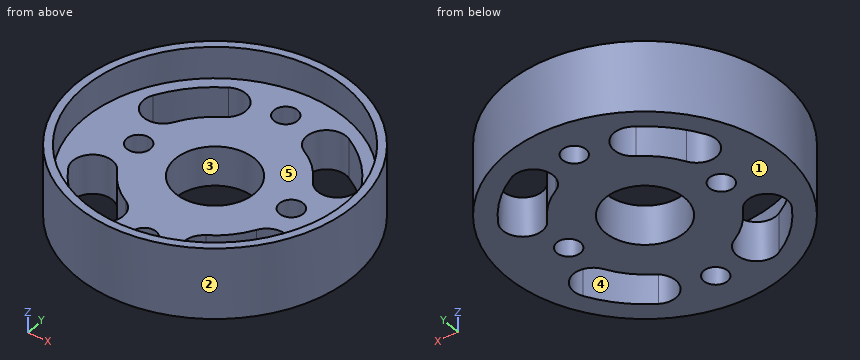
from build123d import *

# Parameters (mm, degrees)
SKETCH1_R           = 17.5
SKETCH1_R_2         = 1.5
SKETCH1_R_3         = 5
BOSS_EXTRUDE1_DEPTH = 5
SKETCH2_R           = 17.5
SKETCH2_R_2         = 16.5
EXTRUDE_THIN1_DEPTH = 4


with BuildPart() as part:
    # Sketch1 → Boss-Extrude1 (new body)
    with BuildSketch(Plane.XY):
        Circle(SKETCH1_R)
        with Locations((0, 12.5)):
            Circle(SKETCH1_R_2, mode=Mode.SUBTRACT)
        with Locations((0, -12.5)):
            Circle(SKETCH1_R_2, mode=Mode.SUBTRACT)
        Circle(SKETCH1_R_3, mode=Mode.SUBTRACT)
        with Locations((9.5, 0)):
            Circle(SKETCH1_R_2, mode=Mode.SUBTRACT)
        with Locations((-9.5, 0)):
            Circle(SKETCH1_R_2, mode=Mode.SUBTRACT)
        with BuildLine():
            ThreePointArc((-8.660254038, -5), (-7.071067812, -7.071067812), (-5, -8.660254038))
            ThreePointArc((-5, -8.660254038), (-4.084936491, -12.075317547), (-7.5, -12.990381057))
            ThreePointArc((-7.5, -12.990381057), (-10.606601718, -10.606601718), (-12.990381057, -7.5))
            ThreePointArc((-12.990381057, -7.5), (-12.075317547, -4.084936491), (-8.660254038, -5))
        make_face(mode=Mode.SUBTRACT)
        with BuildLine():
            ThreePointArc((-5, 8.660254038), (-4.084936491, 12.075317547), (-7.5, 12.990381057))
            ThreePointArc((-7.5, 12.990381057), (-10.606601718, 10.606601718), (-12.990381057, 7.5))
            ThreePointArc((-12.990381057, 7.5), (-12.075317547, 4.084936491), (-8.660254038, 5))
            ThreePointArc((-8.660254038, 5), (-7.071067812, 7.071067812), (-5, 8.660254038))
        make_face(mode=Mode.SUBTRACT)
        with BuildLine():
            ThreePointArc((5, -8.660254038), (4.084936491, -12.075317547), (7.5, -12.990381057))
            ThreePointArc((7.5, -12.990381057), (10.606601718, -10.606601718), (12.990381057, -7.5))
            ThreePointArc((12.990381057, -7.5), (12.075317547, -4.084936491), (8.660254038, -5))
            ThreePointArc((8.660254038, -5), (7.071067812, -7.071067812), (5, -8.660254038))
        make_face(mode=Mode.SUBTRACT)
        with BuildLine():
            ThreePointArc((12.990381057, 7.5), (12.075317547, 4.084936491), (8.660254038, 5))
            ThreePointArc((8.660254038, 5), (7.071067812, 7.071067812), (5, 8.660254038))
            ThreePointArc((5, 8.660254038), (4.084936491, 12.075317547), (7.5, 12.990381057))
            ThreePointArc((7.5, 12.990381057), (10.606601718, 10.606601718), (12.990381057, 7.5))
        make_face(mode=Mode.SUBTRACT)
    extrude(amount=BOSS_EXTRUDE1_DEPTH)

    # Sketch2 → Extrude-Thin1 (add)
    with BuildSketch(Plane.XY.offset(5)):
        Circle(SKETCH2_R)
        Circle(SKETCH2_R_2, mode=Mode.SUBTRACT)
    extrude(amount=EXTRUDE_THIN1_DEPTH)


solid = part.part
Can you work these out from the model? Positions are in its coordinate system, mm. Face numbers are marked on the shaded views. A direction names the side the tool comes from. Round coordinates to 2 decimals unless told otherwise and drop trailing zeros. Loops run counter-clockwise (first coordinate to the right, second up) from the corner with the lowest first, then second, coordinate; pieces in that order, holes last. Notation, with made-up numbers: (9.5, 37) - (63.5, 37) arc R29 cw to (63.5, 74) - close; hole circle Ø6 at (8, -21.5). An arc over 180 degrees is marked (long way). Answer in a Markdown table with one row per item. Add a question column.
Q1. We'd pull the mould along Y, two halves only. Please class the marked faces 1, 2 and 3: pulls with the +Y half, pulls with the -Y half, needs draft (parallel to the pull), parting line crosses it, or undercut.
Q2. Which directions (+Z, -Z, +X, -X, +Y, -Y) give clear straight access to the entire face, cutting with the end or side of a thin tool? Please do the marked faces 4 and 5.
Q3. I want a section at B-B on y = 12.5. List the corners of the cut face in (x, z) for me, and give its area (3 significant figures).
Q4. I need wall thicknesses on L1, parallel to Y at x = 0, z = 2.65; L2, parallel to X at y = 10.5, z = 1.25; L3, parallel to Y at x = 9.5, z = 2.55. Which ranges of each line are inside material? Lowest first, please.
Q5. For pin 1 Ø1.5 at (x, y) = (14, 7) entering from +Z; pin 2 Ø5 at (x, z) = (-6.5, 8) entering from -Y; pin 3 Ø1.5 at (x, z) = (-6.5, 7.5) entering from +Y, each with a flat end and sliding along its axis, tell me the tip position at first contact or that it passes through.
Q6. I want a section at A-A on z = 1.25. Count the separate pieces of the cut face and the enclosed holes in it, and give its area (3 significant figures).
Q7. I want a section at D-D on x = -7. List the corners of the cut face in (y, z) for me, and give its area (3 significant figures).
Q8. I want a section at C-C on x = 0. List the corners of the cut face in (y, z) for me, and give its area (3 significant figures).
A:
| question | item | result |
|---|---|---|
| 1 | face 1 | needs draft |
| 1 | face 2 | parting line crosses it |
| 1 | face 3 | undercut |
| 2 | face 4 | +Z, -Z |
| 2 | face 5 | +Z |
| 3 | outline | (-12.25, 0) - (-8.29, 0) - (-8.29, 5) - (-10.77, 5) - (-10.77, 9) - (-12.25, 9) - close; (-4.39, 0) - (-1.5, 0) - (-1.5, 5) - (-4.39, 5) - close; (1.5, 0) - (4.39, 0) - (4.39, 5) - (1.5, 5) - close; (8.29, 0) - (12.25, 0) - (12.25, 9) - (10.77, 9) - (10.77, 5) - (8.29, 5) - close |
| 3 | area | 80.3 mm^2 |
| 4 | L1 | -17.5 to -14, -11 to -5, 5 to 11, 14 to 17.5 |
| 4 | L2 | -14 to -10.71, -3.77 to 3.77, 10.71 to 14 |
| 4 | L3 | -14.7 to -11.61, -4.13 to -1.5, 1.5 to 4.13, 11.61 to 14.7 |
| 5 | pin 1 | z = 5 |
| 5 | pin 2 | y = -17.04 |
| 5 | pin 3 | y = 16.53 |
| 6 | separate pieces | 1 |
| 6 | enclosed holes | 9 |
| 6 | area | 646 mm^2 |
| 7 | outline | (-16.04, 0) - (-13.21, 0) - (-13.21, 5) - (-14.94, 5) - (-14.94, 9) - (-16.04, 9) - close; (-7.14, 0) - (7.14, 0) - (7.14, 5) - (-7.14, 5) - close; (13.21, 0) - (16.04, 0) - (16.04, 9) - (14.94, 9) - (14.94, 5) - (13.21, 5) - close |
| 7 | area | 108 mm^2 |
| 8 | outline | (-17.5, 0) - (-14, 0) - (-14, 5) - (-16.5, 5) - (-16.5, 9) - (-17.5, 9) - close; (-11, 0) - (-5, 0) - (-5, 5) - (-11, 5) - close; (5, 0) - (11, 0) - (11, 5) - (5, 5) - close; (14, 0) - (17.5, 0) - (17.5, 9) - (16.5, 9) - (16.5, 5) - (14, 5) - close |
| 8 | area | 103 mm^2 |
